```python
from build123d import *

# Parameters (mm, degrees)
SKETCH_1_W          = 130
SKETCH_1_H          = 46
EXTRUDE_1_DEPTH     = 2
SKETCH_3_R          = 2.025
CUT_EXTRUDE_1_DEPTH = 80
SKETCH_4_R          = 2.025
CUT_EXTRUDE_2_DEPTH = 80
CUT_EXTRUDE_3_DEPTH = 10
SKETCH_6_W          = 41.5
SKETCH_6_H          = 24.8
CUT_EXTRUDE_4_DEPTH = 10
CUT_EXTRUDE_5_DEPTH = 10
FILLET_1_R          = 1.6
FILLET_2_R          = 2


with BuildPart() as part:
    # 草图1 → 凸台-拉伸1 (new, symmetric)
    with BuildSketch(Plane.XY):
        Rectangle(SKETCH_1_W, SKETCH_1_H)
    extrude(amount=EXTRUDE_1_DEPTH, both=True)

    # 草图3 → 切除-拉伸1 (cut, symmetric)
    with BuildSketch(Plane(origin=(0, 0, -2), x_dir=(-1, 0, 0), z_dir=(0, 0, -1))):
        with Locations((-60, 19)):
            Circle(SKETCH_3_R)
        with Locations((-60, -19)):
            Circle(SKETCH_3_R)
        with Locations((60, 19)):
            Circle(SKETCH_3_R)
        with Locations((60, -19)):
            Circle(SKETCH_3_R)
    extrude(amount=CUT_EXTRUDE_1_DEPTH, both=True, mode=Mode.SUBTRACT)

    # 草图4 → 切除-拉伸2 (cut, symmetric)
    with BuildSketch(Plane.XY.offset(2)):
        with Locations(Location((47.5, 17.2, 0), (0, 0, 180))):
            Circle(SKETCH_4_R)
        with Locations(Location((47.5, -7.8, 0), (0, 0, 180))):
            Circle(SKETCH_4_R)
        with Locations(Location((-47.5, -7.8, 0), (0, 0, 180))):
            Circle(SKETCH_4_R)
        with Locations(Location((-47.5, 17.2, 0), (0, 0, 180))):
            Circle(SKETCH_4_R)
    extrude(amount=CUT_EXTRUDE_2_DEPTH, both=True, mode=Mode.SUBTRACT)

    # 草图5 → 切除-拉伸3 (cut)
    with BuildSketch(Plane.XY.offset(2)):
        Polygon((-56.971596888, -23), (-44.471596888, -11.8), (44.471596888, -11.8), (56.971596888, -23), align=None)
    extrude(amount=-CUT_EXTRUDE_3_DEPTH, mode=Mode.SUBTRACT)

    # 草图6 → 切除-拉伸4 (cut)
    with BuildSketch(Plane.XY.offset(2)):
        with Locations((-22.75, 5.6)):
            Rectangle(SKETCH_6_W, SKETCH_6_H)
        with Locations((22.75, 5.6)):
            Rectangle(SKETCH_6_W, SKETCH_6_H)
    extrude(amount=-CUT_EXTRUDE_4_DEPTH, mode=Mode.SUBTRACT)

    # 草图7 → 切除-拉伸5 (cut)
    with BuildSketch(Plane.XY.offset(2)):
        Polygon((-60, 14.95874079), (-51.5, 13.73474079), (-51.5, -6.01324065), (-60, -13.62924065), align=None)
        Polygon((51.5, -6.01324065), (60, -13.62924065), (60, 14.95874079), (51.5, 13.73474079), align=None)
    extrude(amount=-CUT_EXTRUDE_5_DEPTH, mode=Mode.SUBTRACT)

    # 圆角1
    fillet_1_edges = [part.edges().sort_by_distance(p)[0] for p in [
        (-2, 18, 0),
        (-2, -6.8, 0),
        (-43.5, -6.8, 0),
        (-43.5, 18, 0),
        (2, 18, 0),
        (43.5, 18, 0),
        (43.5, -6.8, 0),
        (2, -6.8, 0),
        (-60, -13.62924065, 0),
        (-60, 14.95874079, 0),
        (-51.5, 13.73474079, 0),
        (-51.5, -6.01324065, 0),
        (51.5, -6.01324065, 0),
        (51.5, 13.73474079, 0),
        (60, 14.95874079, 0),
        (60, -13.62924065, 0),
    ]]
    fillet(fillet_1_edges, radius=FILLET_1_R)

    # 圆角2
    fillet_2_edges = [part.edges().sort_by_distance(p)[0] for p in [
        (56.971596888, -23, 0),
        (-56.971596888, -23, 0),
        (-44.471596888, -11.8, 0),
        (44.471596888, -11.8, 0),
        (65, -23, 0),
        (-65, -23, 0),
        (-65, 23, 0),
        (65, 23, 0),
    ]]
    fillet(fillet_2_edges, radius=FILLET_2_R)


solid = part.part
```
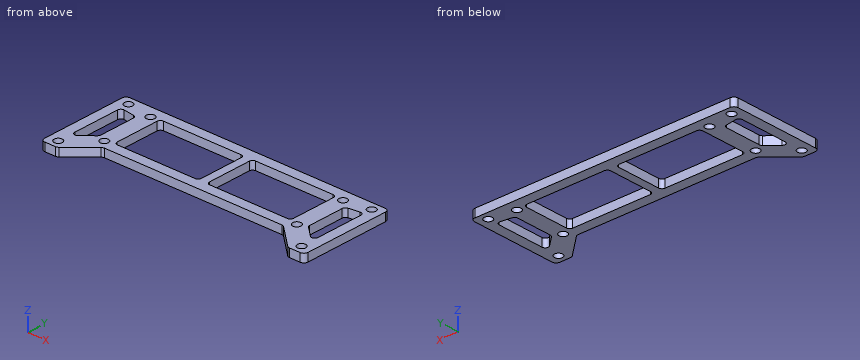
Work out the finished part from the listing and answer in its coordinate system (mm). Round coordinates to 2 decimals unless told otherwise and drop trailing zeros. Write each loop counter-clockwise with the first axis right and the second up, starting at its lowest first coordinate (ties: lowest second). Pieces come first, ordered by that corner, then holes.
1) A cutting plane is placed at A-A on x = -11.5. Determine the outline of the cut face in (y, z).
2) A cutting plane is placed at B-B on y = -15. Determine the outline of the cut face in (x, z), and give its area (3 significant figures).
3) Flat-ended cylindrical pins translate along their axes: P1, Ø2, axis at x = 22.5, z = 0.5, coming from the -Y side; P2, Ø5.5, axis at x = -60, y = -19, coming from the +Z side. Find the tip coordinate at first contact, or state that the pin passes through.
4) A cutting plane is placed at C-C on x = 47.5. Determine the outline of the cut face in (y, z) (3 decimals).
5) A cutting plane is placed at D-D on z = 1.25. Give the number of separate pieces and of enclosed holes in the cut face, and give its area (3 significant figures).
6) Consider probe 1 along X at (y, z) = (5, -1.4); probe 2 along Y at (x, z) = (-7.5, -1.8); probe 3 along Y at (x, z) = (-47.5, 0.55) (3 decimals). Determine where each line is inside the solid, lowest interval first.
Entries:
1. outline: (-11.8, -2) - (-6.8, -2) - (-6.8, 2) - (-11.8, 2) - close; (18, -2) - (23, -2) - (23, 2) - (18, 2) - close
2. outline: (-65, -2) - (-48.04, -2) - (-48.04, 2) - (-65, 2) - close; (48.04, -2) - (65, -2) - (65, 2) - (48.04, 2) - close
2. area: 136 mm2
3. P1: stops at y = -11.8
3. P2: stops at z = 2
4. outline: (-14.513, -2) - (-9.825, -2) - (-9.825, 2) - (-14.513, 2) - close; (-5.775, -2) - (15.175, -2) - (15.175, 2) - (-5.775, 2) - close; (19.225, -2) - (23, -2) - (23, 2) - (19.225, 2) - close
5. separate pieces: 1
5. enclosed holes: 12
5. area: 2,280 mm2
6. probe 1: x = -65 to -60, -51.5 to -43.5, -2 to 2, 43.5 to 51.5, 60 to 65
6. probe 2: y = -11.8 to -6.8, 18 to 23
6. probe 3: y = -14.513 to -9.825, -5.775 to 15.175, 19.225 to 23
